The model under review builds one solid part; all positions refer to its coordinate system, in mm. A direction names the side the tool comes from. Coordinates: 2 decimals unless noted, no trailing zeros. Order: outer loops, then holes, each group sorted by start corner. A loop starts at its lowest first (then second) coordinate and runs counter-clockwise, first axis right, second up. Notation, with made-up numbers: (-33, 8.5) -> (17, 8.5) arc R18 cw to (17, 16.5) -> close; hole circle Ø4 at (74.5, 40). An arc over 180 degrees is marked (long way). Put each result on its own line as item: value.
Autodesk Fusion 360 part; units mm, degrees
sketch "Sketch1" plane through (0, 0, 0) normal (0, 0, 1) x (1, 0, 0)
  line L0 (0, 0) -> (0, 20.32)
  line L1 (3, 20.32) -> (3, 1.5)
  line L2 (20.32, 3) -> (3, 3)
  line L3 (3, 3) -> (3, 1.5)
  line L4 (8.5, 2) -> (8.3025, 2)
  line L5 (20.32, 3) -> (20.32, 0)
  line L6 (0, 20.32) -> (3, 20.32)
  line L7 (22.32, 0) -> (22.32, 1)
  line L8 (19.558, -2) -> (0, -2)
  line L9 (-2, 19.558) -> (-2, -2)
  line L10 (-2, -2) -> (0, -2)
  line L11 (22.32, 0) -> (22.32, -2)
  line L12 (22.32, -2) -> (19.558, -2)
  line L13 (0, 22.32) -> (-2, 22.32)
  line L14 (-2, 22.32) -> (-2, 19.558)
  line L15 (0, 22.32) -> (1, 22.32)
  line L16 (5, 19.558) -> (5, 5)
  line L17 (5, 5) -> (19.558, 5)
  line L18 (1, 22.32) -> (5, 22.32)
  line L19 (5, 22.32) -> (5, 19.558)
  line L20 (19.558, 5) -> (10.5472, 5)
  line L21 (22.32, 1) -> (22.32, 5)
  line L22 (5, 5) -> (22.32, 5)
  line L23 (0, 0) -> (20.32, 0)
  dimension "d30" = 20.32
  dimension "d31" = 20.32
  dimension "d33" = 2
  dimension "d34" = 2
  dimension "d35" = 3
  dimension "d36" = 2
  dimension "d37" = 2
  dimension "d38" = 3
sketch "Sketch2" plane through (0, 0, 0) normal (0, 0, 1) x (-1, 0, 0)
  line L0 (-8.5, 0) -> (0, 0)
  line L1 (0, 0) -> (0, -8.35)
  line L2 (0, -8.35) -> (-1, -8.35)
  line L3 (-1, -8.35) -> (-1, -1)
  line L4 (-1, -1) -> (-8.5, -1)
  line L5 (-9.5, -2) -> (-2, -2)
  line L6 (-2, -9.35) -> (1, -9.35)
  line L7 (1, -9.35) -> (1, -8.35)
  line L8 (-9.5, 0.9516) -> (-9.5, -2)
  line L9 (-3.5, -1) -> (-1, -1)
  line L10 (-1, -1) -> (-1, -4)
  line L11 (-1, -4) -> (-3.5, -4)
  line L12 (-3.5, -4) -> (-3.5, -1)
  line L13 (-3.5, -1) -> (-1, -1)
  line L14 (-1, -4) -> (-1, -1)
  line L15 (-3.5, -1) -> (-1, -1)
  line L16 (1, -8.35) -> (1, 0.9516)
  line L17 (1, 0.9516) -> (-9.5, 0.9516)
  line L18 (-1, -4) -> (-1, -8)
  line L19 (-3.5, -1) -> (-7.5, -1)
  line L20 (-1, -8) -> (-7.5024, -8)
  line L21 (-7.5024, -8) -> (-7.5, -1)
  dimension "d29" = 4
extrude "Extrude3" add sketch "Sketch1" along normal blind 8
extrude "Extrude4" cut sketch "Sketch2" along normal blind 10
sketch "Sketch3" plane through (0, 0, 8) normal (0, 0, 1) x (-1, 0, 0)
  line L0 (-3, -8) -> (-5, -8)
  line L1 (-5, -8) -> (-5, -22.32)
  line L2 (-5, -22.32) -> (2, -22.32)
  line L3 (2, -22.32) -> (2, 2)
  line L4 (2, 2) -> (-22.32, 2)
  line L5 (-22.32, 2) -> (-22.32, -5)
  line L6 (-22.32, -5) -> (-7.5014, -5)
  line L7 (-7.5014, -5) -> (-7.5007, -3)
  line L8 (-7.5007, -3) -> (-20.32, -3)
  line L9 (-20.32, -3) -> (-20.32, 0)
  line L10 (-20.32, 0) -> (0, 0)
  line L11 (0, 0) -> (0, -20.32)
  line L12 (0, -20.32) -> (-3, -20.32)
  line L13 (-3, -20.32) -> (-3, -8)
  line L14 (-5, 0) -> (-5, 0)
  line L15 (-5, 0) -> (-5, -5.022)
  line L16 (-5, -5.022) -> (-5, -5.022)
  line L17 (-5, -5.022) -> (-5, 0)
  line L18 (-22.32, 2) -> (-5, 2)
  line L19 (-5, 2) -> (-5, 2)
  line L20 (-5, 2) -> (-22.32, 2)
  line L21 (-22.32, 2) -> (-22.32, 2)
  line L22 (-5, -5.022) -> (-22.32, -5.022)
  line L23 (-22.32, -5.022) -> (-22.32, -5)
  line L24 (-22.32, -5) -> (-5, -5)
  line L25 (-5, -5) -> (-5, -5.022)
  line L26 (-5, 2) -> (-5, 0)
  line L27 (-22.32, -1.8791) -> (-5, -1.8791)
extrude "Extrude5" cut sketch "Sketch3" against normal blind 8 contours L7 L8 L9 L15 L17 L24 L27 | L5 L6 L7 L8 L9 L24 L27
extrude "Extrude6" add 1 faces at (-1.3333, 13.5467, 8) along direction (0, 0, 1) blind 4
sketch "Sketch4" plane through (0, 0, 12) normal (0, 0, 1) x (-1, 0, 0)
  line L0 (-20.32, 0) -> (0, 0)
  line L1 (-3, -20.32) -> (-3, -8)
  line L2 (-3, -8) -> (-5, -8)
  line L3 (-5, -8) -> (-5, -22.32)
  line L4 (-5, -22.32) -> (2, -22.32)
  line L5 (2, -22.32) -> (2, 2)
  line L6 (2, 2) -> (-22.32, 2)
  line L7 (0, 0) -> (0.25, 0)
  line L8 (0, -20.32) -> (0, 0)
  line L9 (0.25, 0) -> (0.25, -20.5)
  line L10 (0, -20.32) -> (0.25, -20.32)
  line L11 (-22.32, -1.8791) -> (-20.32, -1.8791)
  line L12 (-20.32, -1.8791) -> (-20.32, 0)
  line L13 (-22.32, 2) -> (-22.32, -1.8791)
  dimension "d44" = 0.25
extrude "Extrude7" cut sketch "Sketch4" against normal blind 12
extrude "Extrude8" add 1 faces at (4.3333, 8, 4) along direction (0, -1, 0) blind 4
sketch "Sketch5" plane through (0, 0, 12) normal (0, 0, 1) x (-1, 0, 0)
  line L0 (-20.32, 0) -> (0.25, 0)
  line L1 (0.25, 0) -> (0.25, -20.32)
  line L2 (0.25, -20.32) -> (-3, -20.32)
  line L3 (-3, -20.32) -> (-3, -4)
  line L4 (-3, -4) -> (-5, -4)
  line L5 (-5, -4) -> (-5, -22.32)
  line L6 (-5, -22.32) -> (2, -22.32)
  line L7 (2, -22.32) -> (2, 2)
  line L8 (2, 2) -> (-22.32, 2)
  line L9 (-22.32, 2) -> (-22.32, -1.8791)
  line L10 (-22.32, -1.8791) -> (-20.32, -1.8791)
  line L11 (-20.32, -1.8791) -> (-20.32, 0)
  line L12 (-21.32, -1.8791) -> (-20.32, -1.8791)
  line L13 (-19.32, -1.8791) -> (-19.32, 0)
  line L14 (-22.32, 0.0604) -> (-22.1613, 0)
  line L15 (-22.1613, 0) -> (-19.32, 0)
  line L16 (-22.32, -1.8791) -> (-22.32, 0.0604)
  line L17 (-21.32, -1.8791) -> (-21.32, 0)
  line L18 (-19.32, -1.8791) -> (-19.32, -3.8791)
  line L19 (-19.32, -3.8791) -> (-21.32, -3.8791)
  line L20 (-21.32, -1.8791) -> (-21.32, -3.8791)
  line L21 (-21.32, -1.8791) -> (-22.32, -1.8791)
  line L22 (-21.32, 0) -> (-21.32, 2)
  line L23 (-22.32, 2) -> (-22.32, -1.8791)
  line L24 (-21.32, -1.8791) -> (-22.32, -1.8791)
  line L25 (-21.32, 2) -> (-22.32, 2)
  dimension "d49" = 2
  dimension "d50" = 2
extrude "Extrude9" cut sketch "Sketch5" against normal blind 12 contours L9 L10 L14 L15 L16 L17 L21 L23 L24 | L8 L9 L14 L15 L22 L23 L25
extrude "Extrude10" add sketch "Sketch5" against normal blind 12 contours L0 L10 L11 L12 L13 L15 L18 L19 L20
Item 1: For pin 1 Ø10 at (x, y) = (5.5, 15.5) entering from -Z; pin 2 Ø2 at (x, z) = (14, 6.5) entering from +Y; pin 3 Ø0.6 at (x, z) = (20.5, 7) entering from +Y; pin 4 Ø6 at (y, z) = (7.5, 7) entering from +X, all flat-tipped, find the tip position at first contact; note any pin that passes through.
Answers below:
pin 1: z = 0
pin 2: y = 0
pin 3: y = 3.88
pin 4: x = 5
Item 2: Consider section A-A on y = 19.25. Write out the cut boundary in (x, z), and give its area (3 significant figures).
Answers below:
outline: (-2, 0) -> (-0.25, 0) -> (-0.25, 12) -> (-2, 12) -> close; (3, 0) -> (5, 0) -> (5, 12) -> (3, 12) -> close
area: 45.0 mm^2
Item 3: Consider section C-C on x = 15.5. Write out the cut boundary in (y, z).
Answers below:
outline: (-2, 0) -> (0, 0) -> (0, 12) -> (-2, 12) -> close
Item 4: Mouldability with a two-part tool opening along X and no side actions: class faces 1 (the flat face through (3, 12, 6)), 2 (the flat face through (21.32, 1, 6)), 3 (the flat face through (10, 0, 6)), 4 (the flat face through (20, 3.879, 6)) as +X half, -X half, draft (parallel to the pull), parting line (faces both ways), or undercut.
Answers below:
face 1: undercut
face 2: +X half
face 3: undercut
face 4: draft
Item 5: For line 1 (Y direction, x = 4, z = 5); line 2 (X direction, y = 14.5, z = 6.5); line 3 (X direction, y = 0.25, z = 8.5), list the stretches that pass through material, from the lowest coordinate up. Write a range as from..to.
Answers below:
line 1: -2..0, 4..22.32
line 2: -2..-0.25, 3..5
line 3: -2..-0.25, 19.32..21.32
Item 6: For faces 5 (the flat face through (4, 4, 6)), 6 (the flat face through (19.32, 2, 6)), 7 (the flat face through (5, 13, 6)), 8 (the flat face through (-0.25, 10, 6)), list the 3-axis set-ups (+Z, -Z, +X, -X, +Y, -Y) from which the entire face can be reached by the end or side of a thin tool; tool diameter is ignored.
Answers below:
face 5: +Z, -Z, +X
face 6: +Z, -Z, +Y
face 7: +Z, -Z, +X, +Y
face 8: +Z, -Z
Item 7: Consider section B-B on z = 2.75. Write out the cut boundary in (x, y).
Answers below:
outline: (-2, -2) -> (21.32, -2) -> (21.32, 3.88) -> (19.32, 3.88) -> (19.32, 0) -> (-0.25, 0) -> (-0.25, 20.32) -> (3, 20.32) -> (3, 4) -> (5, 4) -> (5, 22.32) -> (-2, 22.32) -> close
